Part model, mm, in its own coordinate system. A direction names the side the tool comes from. Round coordinates to 2 decimals unless told otherwise and drop trailing zeros. Write each loop counter-clockwise with the first axis right and the second up, starting at its lowest first coordinate (ties: lowest second). Pieces come first, ordered by that corner, then holes. Notation, with made-up numbers: M 63,79.5 L 90,79.5 A25 cw 90,114.5 Z; hole C -2.75,1 d2. An arc over 180 degrees is marked long. Use one line per item in the form item = value. Start each with the question number.
Item 1: Flat gauge pins, fed straight in: pin 1 Ø2 at (x, y) = (7.5, 7) entering from +Z; pin 2 Ø1.3 at (x, y) = (5, -5.5) entering from -Z; pin 3 Ø1.1 at (x, y) = (0.5, -8.5) entering from +Z. Where does each tip first touch, or does it go through?
Item 2: Cut at D-D, the plane x = 5.5. Give the cut face in (y, z).
Item 3: Cut at C-C, the plane z = 2.25. Give the cut face in (x, y), then the cut area to 3 significant figures.
Item 4: Mould opens along Y. For faces 1 (the face through (-7, -7, 11.7)), 2 (the face through (-8.51, 8.46, 4.68)), 3 (the face through (-9, 9, 9.5)), 4 (the face through (-9.53, -9.5, 12.39)) say: +Y half, -Y half, draft (parallel to the pull), parting line (faces both ways), or undercut.
Item 5: Which spindle directions (+Z, -Z, +X, -X, +Y, -Y) get a long thin tool onto all of the face, cutting with end or side? Do faces 5 (the face through (9.6, 7, 12)), 6 (the face through (-7.85, -9.68, 13.86)), 7 (the face through (-9, 0, 6.7)), 8 (the face through (9.304, 1.335, 4.471)), 9 (the face through (-5.7, -5.7, 8.1)). Say none if no direction does.
Item 6: Cut at A-A, the plane z = 9. Give the cut face in (x, y), then the cut area to 3 significant figures.
Item 7: Cut at B-B, the plane y = 0. Give the cut face in (x, z), then the cut area to 3 significant figures.
Item 8: Probe L1, parallel to X at y = 0, z = 2.25; L2, parallel to Z at x = 7.75, y = -5.75. List the from-to ranges inside material, lowest first.
from build123d import *

# Parameters (mm, degrees)
SKETCH_W        = 20.2
SKETCH_H        = 20.2
PAD_DEPTH       = 15.2
POCKET_DEPTH    = 3.5
POCKET001_DEPTH = 20.201
POCKET002_DEPTH = 20.201
SKETCH008_R     = 8.6
POCKET003_DEPTH = 8.1
SKETCH009_W     = 7
SKETCH009_H     = 5
POCKET004_DEPTH = 20.201
SKETCH010_W     = 7
SKETCH010_H     = 5
POCKET005_DEPTH = 20.201
SKETCH011_R     = 20
SKETCH011_R_2   = 12
POCKET006_DEPTH = 9.5
SKETCH012_R     = 7
POCKET007_DEPTH = 7.101
SKETCH013_R     = 1.4
POCKET008_DEPTH = 3
FILLET_R        = 2


with BuildPart() as part:
    # Sketch → Pad (new body)
    with BuildSketch(Plane.XY):
        Rectangle(SKETCH_W, SKETCH_H)
    extrude(amount=PAD_DEPTH)

    # Sketch004 → Pocket (cut)
    with BuildSketch(Plane.XY.offset(15.2)):
        Polygon((9.6, 7.65), (7.65, 9.6), (-7.65, 9.6), (-9.6, 7.65), (-9.6, -7.65), (-7.65, -9.6), (7.65, -9.6), (9.6, -7.65), align=None)
    extrude(amount=-POCKET_DEPTH, mode=Mode.SUBTRACT)

    # Sketch006 → Pocket001 (cut, through all)
    with BuildSketch(Plane(origin=(-10.1, 0, 0), x_dir=(0, -1, 0), z_dir=(-1, 0, 0))):
        Polygon((-9, 15.2), (-6, 11.7), (6, 11.7), (9, 15.2), align=None)
    extrude(amount=-POCKET001_DEPTH, mode=Mode.SUBTRACT)

    # Sketch007 → Pocket002 (cut, through all)
    with BuildSketch(Plane(origin=(0, 10.1, 0), x_dir=(-1, 0, 0), z_dir=(0, 1, 0))):
        Polygon((-9, 15.2), (9, 15.2), (6, 11.7), (-6, 11.7), align=None)
    extrude(amount=-POCKET002_DEPTH, mode=Mode.SUBTRACT)

    # Sketch008 → Pocket003 (cut)
    with BuildSketch(Plane(origin=(0, 0, 0), x_dir=(1, 0, 0), z_dir=(0, 0, -1))):
        Circle(SKETCH008_R)
    extrude(amount=-POCKET003_DEPTH, mode=Mode.SUBTRACT)

    # Sketch009 → Pocket004 (cut, through all)
    with BuildSketch(Plane.YZ.offset(10.1)):
        with Locations((0, 9.2)):
            Rectangle(SKETCH009_W, SKETCH009_H)
    extrude(amount=-POCKET004_DEPTH, mode=Mode.SUBTRACT)

    # Sketch010 → Pocket005 (cut, through all)
    with BuildSketch(Plane.XZ.offset(10.1)):
        with Locations((0, 9.2)):
            Rectangle(SKETCH010_W, SKETCH010_H)
    extrude(amount=-POCKET005_DEPTH, mode=Mode.SUBTRACT)

    # Sketch011 → Pocket006 (cut)
    with BuildSketch(Plane(origin=(0, 0, 0), x_dir=(1, 0, 0), z_dir=(0, 0, -1))):
        Circle(SKETCH011_R)
        Circle(SKETCH011_R_2, mode=Mode.SUBTRACT)
    extrude(amount=-POCKET006_DEPTH, mode=Mode.SUBTRACT)

    # Sketch012 → Pocket007 (cut, through all)
    with BuildSketch(Plane(origin=(0, 0, 8.1), x_dir=(1, 0, 0), z_dir=(0, 0, -1))):
        Circle(SKETCH012_R)
    extrude(amount=-POCKET007_DEPTH, mode=Mode.SUBTRACT)

    # Sketch013 → Pocket008 (cut)
    with BuildSketch(Plane.YZ.offset(10.1)):
        with Locations((0, 4.05)):
            Circle(SKETCH013_R)
    extrude(amount=-POCKET008_DEPTH, mode=Mode.SUBTRACT)

    # Fillet
    fillet_edges = [part.edges().sort_by_distance(p)[0] for p in [
        (10.1, 10.1, 12.35),
        (-10.1, 10.1, 12.35),
        (10.1, -10.1, 12.35),
        (-10.1, -10.1, 12.35),
    ]]
    fillet(fillet_edges, radius=FILLET_R)


solid = part.part
Model answer:
q1.pin_1 = 11.7
q1.pin_2 = 8.1
q1.pin_3 = 6.7
q2.outline = M -10.1,0 L -6.61,0 L -6.61,8.1 L -4.33,8.1 L -4.33,11.7 L -10.1,11.7 Z; M 4.33,8.1 L 6.61,8.1 L 6.61,0 L 10.1,0 L 10.1,11.7 L 4.33,11.7 Z
q3.outline = M -10.1,-6.48 A12 ccw -6.48,-10.1 L 6.48,-10.1 A12 ccw 10.1,-6.48 L 10.1,6.48 A12 ccw 6.48,10.1 L -6.48,10.1 A12 ccw -10.1,6.48 Z; hole C 0,0 d17.2
q3.area = 153 mm²
q4.face_1 = undercut
q4.face_2 = +Y half
q4.face_3 = draft
q4.face_4 = -Y half
q5.face_5 = +Z
q5.face_6 = +Z, +Y, -Y
q5.face_7 = +Z, +X, -X
q5.face_8 = +X
q5.face_9 = -Z
q6.outline = M -10.1,-6.48 A12 ccw -6.48,-10.1 L -3.5,-10.1 L -3.5,-6.06 A7 cw -6.06,-3.5 L -10.1,-3.5 Z; M -10.1,3.5 L -6.06,3.5 A7 cw -3.5,6.06 L -3.5,10.1 L -6.48,10.1 A12 ccw -10.1,6.48 Z; M 3.5,-10.1 L 6.48,-10.1 A12 ccw 10.1,-6.48 L 10.1,-3.5 L 6.06,-3.5 A7 cw 3.5,-6.06 Z; M 3.5,6.06 A7 cw 6.06,3.5 L 10.1,3.5 L 10.1,6.48 A12 ccw 6.48,10.1 L 3.5,10.1 Z
q6.area = 136 mm²
q7.outline = M -10.1,0 L -8.6,0 L -8.6,6.7 L -10.1,6.7 Z; M 8.6,0 L 10.1,0 L 10.1,2.65 L 8.6,2.65 Z; M 8.6,5.45 L 10.1,5.45 L 10.1,6.7 L 8.6,6.7 Z
q7.area = 15.9 mm²
q8.L1 = -10.1 to -8.6, 8.6 to 10.1
q8.L2 = 0 to 11.7
